Job drawing, mm, ordinate dimensions from the low corner. One solid piece. Coordinates: 2 decimals unless noted, no trailing zeros. Order: outer loops, then holes, each group sorted by start corner. A loop starts at its lowest first (then second) coordinate and runs counter-clockwise, first axis right, second up. Notation, with made-up numbers: (6.25, -38.5) - (18.25, -38.5) arc R10 ccw to (18.25, -29.5) - close; hole circle Ø11 at (76.25, 7.25). An arc over 180 degrees is marked (long way). Return JSON: item names as keys, results as strings.
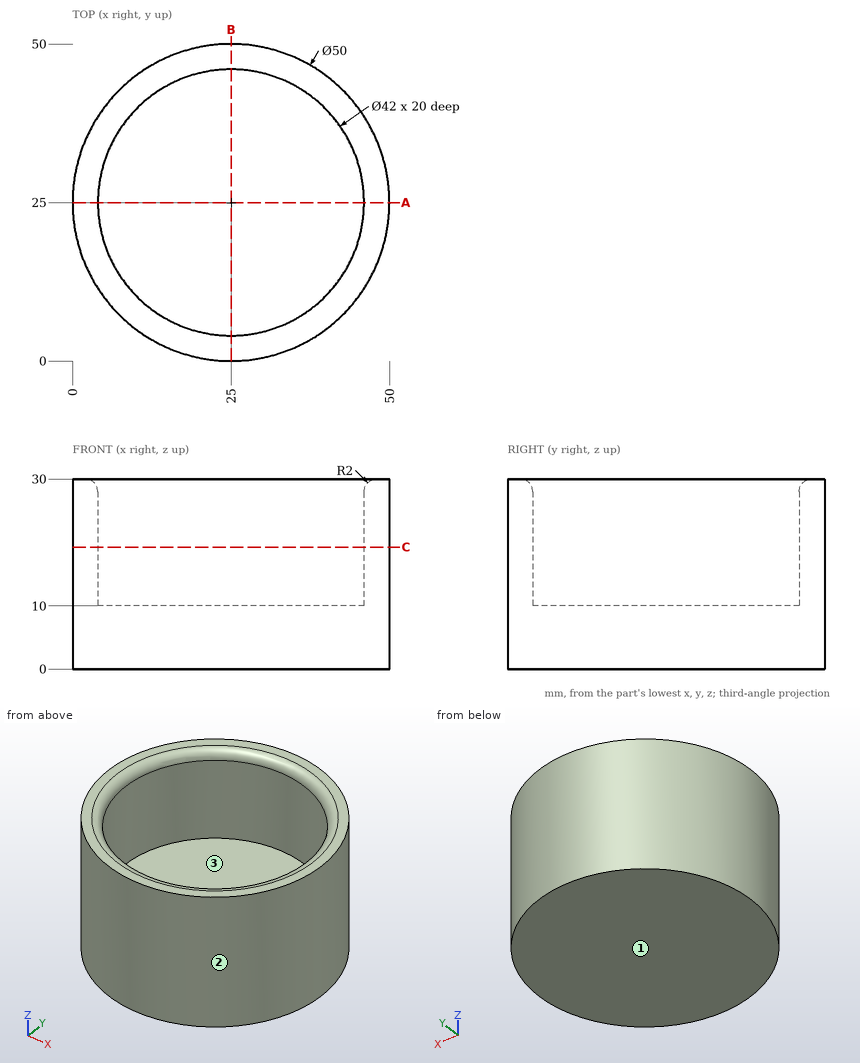
1. Cut at C-C on z = 19.25. Give the cut face in (x, y), plus the area to 3 significant figures.
Check values:
{"outline": "circle Ø50 at (25, 25); hole circle Ø42 at (25, 25)", "area": "578 mm²"}
2. Mould opens along Y. For the marked faces 1, 2 and 3 say: pulls with the +Y half, pulls with the -Y half, needs draft (parallel to the pull), parting line crosses it, or undercut.
Check values:
{"face 1": "needs draft", "face 2": "parting line crosses it", "face 3": "undercut"}
3. Cut at A-A on y = 25. Give the cut face in (x, z), plus the area to 3 significant figures.
Check values:
{"outline": "(0, 0) - (50, 0) - (50, 30) - (48, 30) arc R2 ccw to (46, 28) - (46, 10) - (4, 10) - (4, 28) arc R2 ccw to (2, 30) - (0, 30) - close", "area": "658 mm²"}
4. Drop flat-ended pins along their axis: pin 1 (21 mm diameter, centred on x = 34.5, y = 30, fed in from +Z); pin 2 (5 mm diameter, centred on x = 31, z = 19, fed in from +Y); pin 3 (5 mm diameter, centred on x = 33.5, z = 7.5, fed in from -Y). Give the stop position or say it passes through.
Check values:
{"pin 1": "z = 28.94", "pin 2": "y = 49.75", "pin 3": "y = 0.73"}
5. Probe L1, parallel to Y at x = 25, z = 17.25; L2, parallel to Z at x = 35, y = 14.5; L3, parallel to Y at x = 42, z = 15. List the from-to ranges inside material, lowest first.
Check values:
{"L1": "0 to 4, 46 to 50", "L2": "0 to 10", "L3": "6.67 to 12.67, 37.33 to 43.33"}
